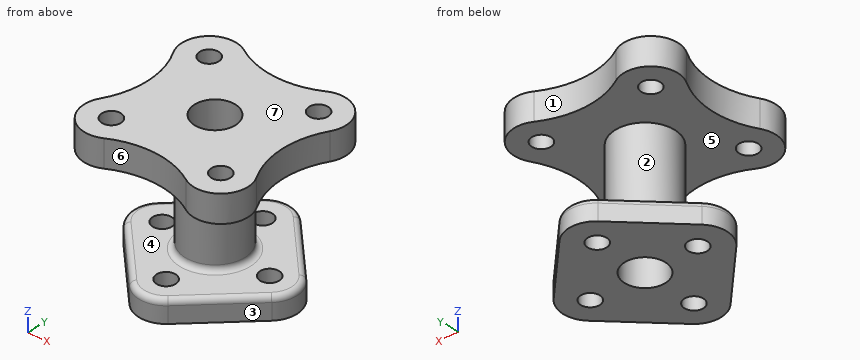
```python
from build123d import *

# Parameters (mm, degrees)
EXTRUDE_1_DEPTH     = 12.7
SKETCH_2_R          = 13.97
EXTRUDE_2_DEPTH     = 43.18
EXTRUDE_3_DEPTH     = 10.16
SKETCH_5_R          = 9.525
CUT_EXTRUDE_1_DEPTH = 86.232045617
CUT_EXTRUDE_2_REACH = 87.232
SKETCH_6_R          = 4.445
CUT_EXTRUDE_3_REACH = 79.626
SKETCH_7_R          = 4.445
FILLET_1_R          = 2.54


with BuildPart() as part:
    # 스케치1 → 보스-돌출1 (new body)
    with BuildSketch(Plane.XY):
        with BuildLine():
            ThreePointArc((-19.05, 36.398522628), (-34.380256121, 34.380256121), (-36.398522628, 19.05))
            ThreePointArc((-36.398522628, 19.05), (-31.294090512, 0), (-36.398522628, -19.05))
            ThreePointArc((-36.398522628, -19.05), (-34.380256121, -34.380256121), (-19.05, -36.398522628))
            ThreePointArc((-19.05, -36.398522628), (0, -31.294090512), (19.05, -36.398522628))
            ThreePointArc((19.05, -36.398522628), (34.380256121, -34.380256121), (36.398522628, -19.05))
            ThreePointArc((36.398522628, -19.05), (31.294090512, 0), (36.398522628, 19.05))
            ThreePointArc((36.398522628, 19.05), (34.380256121, 34.380256121), (19.05, 36.398522628))
            ThreePointArc((19.05, 36.398522628), (0, 31.294090512), (-19.05, 36.398522628))
        make_face()
    extrude(amount=-EXTRUDE_1_DEPTH)

    # 스케치2 → 보스-돌출2 (add)
    with BuildSketch(Plane(origin=(0, 0, -12.7), x_dir=(-1, 0, 0), z_dir=(0, 0, -1))):
        Circle(SKETCH_2_R)
    extrude(amount=EXTRUDE_2_DEPTH)

    # 스케치4 → 보스-돌출3 (add)
    with BuildSketch(Plane(origin=(0, 0, -55.88), x_dir=(-1, 0, 0), z_dir=(0, 0, -1))):
        with BuildLine():
            Line((-34.380256121, 8.980256121), (-8.980256121, 34.380256121))
            ThreePointArc((-8.980256121, 34.380256121), (0, 38.1), (8.980256121, 34.380256121))
            Line((8.980256121, 34.380256121), (34.380256121, 8.980256121))
            ThreePointArc((34.380256121, 8.980256121), (38.1, 0), (34.380256121, -8.980256121))
            Line((34.380256121, -8.980256121), (8.980256121, -34.380256121))
            ThreePointArc((8.980256121, -34.380256121), (0, -38.1), (-8.980256121, -34.380256121))
            Line((-8.980256121, -34.380256121), (-34.380256121, -8.980256121))
            ThreePointArc((-34.380256121, -8.980256121), (-38.1, 0), (-34.380256121, 8.980256121))
        make_face()
    extrude(amount=EXTRUDE_3_DEPTH)

    # 스케치5 → 컷-돌출1 (cut, through all)
    with BuildSketch(Plane.XY):
        Circle(SKETCH_5_R)
    extrude(amount=-CUT_EXTRUDE_1_DEPTH, mode=Mode.SUBTRACT)

    # 스케치6 → 컷-돌출2 (cut, up to next)
    with BuildSketch(Plane.XY, mode=Mode.PRIVATE) as cut_extrude_2_sk1:
        with Locations((-25.4, 25.4)):
            Circle(SKETCH_6_R)
    cut_extrude_2_tool1 = extrude(cut_extrude_2_sk1.sketch, amount=-CUT_EXTRUDE_2_REACH, mode=Mode.PRIVATE) & part.part
    # 스케치6 → 컷-돌출2 (cut, up to next)
    with BuildSketch(Plane.XY, mode=Mode.PRIVATE) as cut_extrude_2_sk2:
        with Locations((-25.4, -25.4)):
            Circle(SKETCH_6_R)
    cut_extrude_2_tool2 = extrude(cut_extrude_2_sk2.sketch, amount=-CUT_EXTRUDE_2_REACH, mode=Mode.PRIVATE) & part.part
    # 스케치6 → 컷-돌출2 (cut, up to next)
    with BuildSketch(Plane.XY, mode=Mode.PRIVATE) as cut_extrude_2_sk3:
        with Locations((25.4, -25.4)):
            Circle(SKETCH_6_R)
    cut_extrude_2_tool3 = extrude(cut_extrude_2_sk3.sketch, amount=-CUT_EXTRUDE_2_REACH, mode=Mode.PRIVATE) & part.part
    # 스케치6 → 컷-돌출2 (cut, up to next)
    with BuildSketch(Plane.XY, mode=Mode.PRIVATE) as cut_extrude_2_sk4:
        with Locations((25.4, 25.4)):
            Circle(SKETCH_6_R)
    cut_extrude_2_tool4 = extrude(cut_extrude_2_sk4.sketch, amount=-CUT_EXTRUDE_2_REACH, mode=Mode.PRIVATE) & part.part
    add(cut_extrude_2_tool1.solids().sort_by_distance((-25.4, 25.4, 0))[0], mode=Mode.SUBTRACT)
    add(cut_extrude_2_tool2.solids().sort_by_distance((-25.4, -25.4, 0))[0], mode=Mode.SUBTRACT)
    add(cut_extrude_2_tool3.solids().sort_by_distance((25.4, -25.4, 0))[0], mode=Mode.SUBTRACT)
    add(cut_extrude_2_tool4.solids().sort_by_distance((25.4, 25.4, 0))[0], mode=Mode.SUBTRACT)

    # 스케치7 → 컷-돌출3 (cut, up to next)
    with BuildSketch(Plane.XY.offset(-55.88), mode=Mode.PRIVATE) as cut_extrude_3_sk1:
        with Locations((0, 24.823944536)):
            Circle(SKETCH_7_R)
    cut_extrude_3_tool1 = extrude(cut_extrude_3_sk1.sketch, amount=-CUT_EXTRUDE_3_REACH, mode=Mode.PRIVATE) & part.part
    # 스케치7 → 컷-돌출3 (cut, up to next)
    with BuildSketch(Plane.XY.offset(-55.88), mode=Mode.PRIVATE) as cut_extrude_3_sk2:
        with Locations((25.4, 0)):
            Circle(SKETCH_7_R)
    cut_extrude_3_tool2 = extrude(cut_extrude_3_sk2.sketch, amount=-CUT_EXTRUDE_3_REACH, mode=Mode.PRIVATE) & part.part
    # 스케치7 → 컷-돌출3 (cut, up to next)
    with BuildSketch(Plane.XY.offset(-55.88), mode=Mode.PRIVATE) as cut_extrude_3_sk3:
        with Locations((0, -25.4)):
            Circle(SKETCH_7_R)
    cut_extrude_3_tool3 = extrude(cut_extrude_3_sk3.sketch, amount=-CUT_EXTRUDE_3_REACH, mode=Mode.PRIVATE) & part.part
    # 스케치7 → 컷-돌출3 (cut, up to next)
    with BuildSketch(Plane.XY.offset(-55.88), mode=Mode.PRIVATE) as cut_extrude_3_sk4:
        with Locations((-24.501420948, 0)):
            Circle(SKETCH_7_R)
    cut_extrude_3_tool4 = extrude(cut_extrude_3_sk4.sketch, amount=-CUT_EXTRUDE_3_REACH, mode=Mode.PRIVATE) & part.part
    add(cut_extrude_3_tool1.solids().sort_by_distance((0, 24.823945, -55.88))[0], mode=Mode.SUBTRACT)
    add(cut_extrude_3_tool2.solids().sort_by_distance((25.4, 0, -55.88))[0], mode=Mode.SUBTRACT)
    add(cut_extrude_3_tool3.solids().sort_by_distance((0, -25.4, -55.88))[0], mode=Mode.SUBTRACT)
    add(cut_extrude_3_tool4.solids().sort_by_distance((-24.501421, 0, -55.88))[0], mode=Mode.SUBTRACT)

    # 필렛1
    fillet_1_edges = [part.edges().sort_by_distance(p)[0] for p in [
        (13.97, 0, -55.88),
        (-38.1, 0, -55.88),
        (-21.680256121, 21.680256121, -55.88),
        (0, 38.1, -55.88),
        (21.680256121, 21.680256121, -55.88),
        (38.1, 0, -55.88),
        (21.680256121, -21.680256121, -55.88),
        (0, -38.1, -55.88),
        (-21.680256121, -21.680256121, -55.88),
    ]]
    fillet(fillet_1_edges, radius=FILLET_1_R)


solid = part.part
```
Model file for the job. Use its own axes, mm. Face numbers are marked on the shaded views. A direction names the side the tool comes from. Round coordinates to 2 decimals unless told otherwise and drop trailing zeros. Loops run counter-clockwise (first coordinate to the right, second up) from the corner with the lowest first, then second, coordinate; pieces in that order, holes last. Notation, with made-up numbers: M 78.5,55.5 L 129.5,55.5 A23 ccw 129.5,79.5 Z; hole C 46,42.25 d9. An arc over 180 degrees is marked long. Put each result on its own line as item: value. Start each with the question number.
Item 1: Cut at C-C (z = -9). List the corners of the cut face in (x, y) (3 decimals), then the cut area to 3 significant figures.
Item 2: Drill centre lines: line 1 along Y through (x, z) = (25.4, -8) (3 decimals); line 2 along X through (y, z) = (-25, -7); line 3 along Z through (x, y) = (20.5, 10). Where is each one in solid material? Low to high.
Item 3: Cut at A-A (x = 0). List the corners of the cut face in (y, z) (3 decimals), then the cut area to 3 significant figures.
Item 4: Drop flat-ended pins along their axis: P1, Ø8, axis at y = -28, z = -59, coming from the +X side; P2, Ø7, axis at x = -24.5, y = 0, coming from the -Z side; P3, Ø2, axis at y = -9.5, z = -54.5, coming from the -X side. Give the stop position or say it passes through.
Item 5: Cut at D-D (z = -45.5). List the corners of the cut face in (x, y) (3 decimals).
Item 6: Mould opens along Z. For the marked faces 4, 5, 6 and 7 say: released by +Z, released by -Z, zero draft, split by the parting line, or undercut.
Item 7: 3-axis set-ups, long thin cutter, end or side, ignore diameter. For the marked faces 1, 2 and 3: which of +Z, -Z, +X, -X, +Y, -Y reach the whole face in a straight line?
Item 8: Cut at B-B (y = 0). List the corners of the cut face in (x, z) (3 decimals).
Answer block:
1. outline: M -36.399,-19.05 A12.7 ccw -19.05,-36.399 A38.1 cw 19.05,-36.399 A12.7 ccw 36.399,-19.05 A38.1 cw 36.399,19.05 A12.7 ccw 19.05,36.399 A38.1 cw -19.05,36.399 A12.7 ccw -36.399,19.05 A38.1 cw Z; hole C -25.4,-25.4 d8.89; hole C -25.4,25.4 d8.89; hole C 0,0 d19.05; hole C 25.4,-25.4 d8.89; hole C 25.4,25.4 d8.89
1. area: 4,320 mm2
2. line 1: -38.1 to -29.845, -20.955 to 20.955, 29.845 to 38.1
2. line 2: -38.09 to -29.83, -20.97 to 20.97, 29.83 to 38.09
2. line 3: -66.04 to -55.88, -12.7 to 0
3. outline: M -38.1,-66.04 L -29.845,-66.04 L -29.845,-55.88 L -35.56,-55.88 A2.54 ccw -38.1,-58.42 Z; M -31.294,-12.7 L -13.97,-12.7 L -13.97,-53.34 A2.54 cw -16.51,-55.88 L -20.955,-55.88 L -20.955,-66.04 L -9.525,-66.04 L -9.525,0 L -31.294,0 Z; M 9.525,-66.04 L 20.379,-66.04 L 20.379,-55.88 L 16.51,-55.88 A2.54 cw 13.97,-53.34 L 13.97,-12.7 L 31.294,-12.7 L 31.294,0 L 9.525,0 Z; M 29.269,-66.04 L 38.1,-66.04 L 38.1,-58.42 A2.54 ccw 35.56,-55.88 L 29.269,-55.88 Z
3. area: 1,340 mm2
4. P1: x = 19.36
4. P2: z = -12.7
4. P3: x = -11.98
5. outline: C 0,0 d27.94; hole C 0,0 d19.05
6. face 4: undercut
6. face 5: undercut
6. face 6: zero draft
6. face 7: released by +Z
7. face 1: +Z, +Y
7. face 2: none
7. face 3: -Z, +X, -Y
8. outline: M -38.1,-66.04 L -28.946,-66.04 L -28.946,-55.88 L -35.56,-55.88 A2.54 ccw -38.1,-58.42 Z; M -31.294,-12.7 L -13.97,-12.7 L -13.97,-53.34 A2.54 cw -16.51,-55.88 L -20.056,-55.88 L -20.056,-66.04 L -9.525,-66.04 L -9.525,0 L -31.294,0 Z; M 9.525,-66.04 L 20.955,-66.04 L 20.955,-55.88 L 16.51,-55.88 A2.54 cw 13.97,-53.34 L 13.97,-12.7 L 31.294,-12.7 L 31.294,0 L 9.525,0 Z; M 29.845,-66.04 L 38.1,-66.04 L 38.1,-58.42 A2.54 ccw 35.56,-55.88 L 29.845,-55.88 Z
